```python
from build123d import *

# Parameters (mm, degrees)
SKETCH1_W           = 40
SKETCH1_H           = 40
BOSS_EXTRUDE1_DEPTH = 40
CUT_EXTRUDE1_DEPTH  = 40
CUT_EXTRUDE2_DEPTH  = 40


with BuildPart() as part:
    # Sketch1 → Boss-Extrude1 (new body)
    with BuildSketch(Plane.XY):
        with Locations((20, 20)):
            Rectangle(SKETCH1_W, SKETCH1_H)
    extrude(amount=BOSS_EXTRUDE1_DEPTH)

    # Sketch2 → Cut-Extrude1 (cut)
    with BuildSketch(Plane.XY.offset(40)):
        Polygon((0, 0), (20, 40), (0, 40), align=None)
    extrude(amount=-CUT_EXTRUDE1_DEPTH, mode=Mode.SUBTRACT)

    # Sketch3 → Cut-Extrude2 (cut)
    with BuildSketch(Plane.XZ):
        Polygon((40, 20), (20, 20), (0, 40), (40, 40), align=None)
    extrude(amount=-CUT_EXTRUDE2_DEPTH, mode=Mode.SUBTRACT)


solid = part.part
```
Here's how the part is built. I have some questions about the finished solid (model axes, mm). A direction names the side the tool comes from. Coordinates: 2 decimals unless noted, no trailing zeros. Loops run counter-clockwise (first coordinate to the right, second up) from the corner with the lowest first, then second, coordinate; pieces in that order, holes last. Notation, with made-up numbers: (28.5, 21.25) - (33.5, 21.25) arc R16 cw to (33.5, 37.25) - close; hole circle Ø10 at (11.5, -15). An arc over 180 degrees is marked (long way). Return JSON: item names as keys, results as strings. Group by question number.
Item 1: I need wall thicknesses on line 1 (Z direction, x = 36, y = 23.5); line 2 (Y direction, x = 13.5, z = 24); line 3 (Z direction, x = 15, y = 8). Which ranges of each line are inside material? Lowest first, please. Write a range as from..to.
Item 2: If we section it at B-B on z = 37.5: Write out the boundary of the cut face in (x, y), and give its area (3 significant figures).
Item 3: If we section it at C-C on x = 3: Write out the boundary of the cut face in (y, z), and give its area (3 significant figures).
Item 4: Will these pins go through, and if not, where does the flat tip stop? P1, Ø3, axis at x = 15, y = 6.5, coming from the +Z side; P2, Ø4, axis at x = 24, y = 30.5, coming from the +Z side; P3, Ø1.5, axis at x = 16, y = 20.5, coming from the +Z side.
Item 5: If we section it at A-A on y = 8.5: Write out the boundary of the cut face in (x, z).
Item 6: On a 3-axis mill with a long thin cutter (end or side, diameter ignored), from which of +Z, -Z, +X, -X, +Y, -Y can I reach the whole of each face in a straight line? I mean faces 1 (the face through (30, 40, 10)), 2 (the face through (30, 20, 20)). Say none if no direction works.
Item 7: If we section it at D-D on y = 26: Write out the boundary of the cut face in (x, z), and give its area (4 significant figures).
Calculated:
{
 "1": {"line 1": "z = 0..20", "line 2": "y = 0..27", "line 3": "z = 0..25"},
 "2": {"outline": "(0, 0) - (2.5, 0) - (2.5, 5) - close", "area": "6.25 mm^2"},
 "3": {"outline": "(0, 0) - (6, 0) - (6, 37) - (0, 37) - close", "area": "222 mm^2"},
 "4": {"P1": "stops at z = 26.5", "P2": "stops at z = 20", "P3": "stops at z = 24.75"},
 "5": {"outline": "(4.25, 0) - (40, 0) - (40, 20) - (20, 20) - (4.25, 35.75) - close"},
 "6": {"face 1": "+Z, -Z, +X, -X, +Y", "face 2": "+Z, +X, +Y, -Y"},
 "7": {"outline": "(13, 0) - (40, 0) - (40, 20) - (20, 20) - (13, 27) - close", "area": "564.5 mm^2"}
}
